from build123d import *

# Parameters (mm, degrees)
F0_W         = 156
F0_H         = 10
F0_R         = 1.5
F1_DEPTH     = 8
F2_T1_DEPTH  = 4
F2_T3_DEPTH  = 18
F2_T5_DEPTH  = 159
F2_T7_DEPTH  = 13
F2_S11_W     = 2
F2_S11_H     = 2
F2_T12_DEPTH = 2
F2_S17_W     = 2
F2_S17_H     = 2
F2_T18_DEPTH = 2
F3_T1_DEPTH  = 11
F3_T3_DEPTH  = 4
F3_T5_DEPTH  = 157
F3_S9_W      = 2.04
F3_S9_H      = 2.04
F3_T10_DEPTH = 2.04
F3_S15_W     = 2.04
F3_S15_H     = 2.04
F3_T16_DEPTH = 2.04


# Not quite as in the source:
# - a fillet or chamfer that OpenCascade refuses, or shapes differently, is made with other operations: its cross-section is extruded or revolved along the edge and cut away or added


with BuildPart() as f1:
    # F0 (on Front) → F1 (new body)
    with BuildSketch(Plane.XZ):
        with Locations((-25, 5)):
            Rectangle(F0_W, F0_H)
        with Locations((-100, 5)):
            Circle(F0_R, mode=Mode.SUBTRACT)
        with Locations((50, 5)):
            Circle(F0_R, mode=Mode.SUBTRACT)
    extrude(amount=F1_DEPTH)

    # F2: fillet of radius 2 on 7 edges, made by hand

    # F2_s2 → F2_t1 (cut)
    with BuildSketch(Plane.XZ.offset(2)):
        with BuildLine():
            ThreePointArc((53, 8), (52.4142135624, 9.4142135624), (51, 10))
            Line((51, 10), (53, 10))
            Line((53, 10), (53, 8))
        make_face()
    extrude(amount=F2_T1_DEPTH, mode=Mode.SUBTRACT)

    # F2_s4 → F2_t3 (cut)
    with BuildSketch(Plane.XZ.offset(-5)):
        with BuildLine():
            ThreePointArc((-103, 8), (-102.4142135624, 9.4142135624), (-101, 10))
            Line((-101, 10), (-103, 10))
            Line((-103, 10), (-103, 8))
        make_face()
        with BuildLine():
            ThreePointArc((51, 0), (52.4142135624, 0.5857864376), (53, 2))
            Line((53, 2), (53, 0))
            Line((53, 0), (51, 0))
        make_face()
    extrude(amount=F2_T3_DEPTH, mode=Mode.SUBTRACT)

    # F2_s6 → F2_t5 (cut)
    with BuildSketch(Plane.YZ.offset(-108)):
        with BuildLine():
            ThreePointArc((-2, 10), (-0.5857864376, 9.4142135624), (0, 8))
            Line((0, 8), (0, 10))
            Line((0, 10), (-2, 10))
        make_face()
        with BuildLine():
            ThreePointArc((-6, 10), (-7.4142135624, 9.4142135624), (-8, 8))
            Line((-8, 8), (-8, 10))
            Line((-8, 10), (-6, 10))
        make_face()
    extrude(amount=F2_T5_DEPTH, mode=Mode.SUBTRACT)

    # F2_s8 → F2_t7 (cut)
    with BuildSketch(Plane.XY.offset(-5)):
        with BuildLine():
            ThreePointArc((53, -2), (52.4142135624, -0.5857864376), (51, 0))
            Line((51, 0), (53, 0))
            Line((53, 0), (53, -2))
        make_face()
        with BuildLine():
            ThreePointArc((53, -6), (52.4142135624, -7.4142135624), (51, -8))
            Line((51, -8), (53, -8))
            Line((53, -8), (53, -6))
        make_face()
    extrude(amount=F2_T7_DEPTH, mode=Mode.SUBTRACT)


with BuildPart() as f2_tool10:
    # F2_s11 → F2_t12 (new body)
    with BuildSketch(Plane.YZ.offset(51)):
        with Locations((-1, 9)):
            Rectangle(F2_S11_W, F2_S11_H)
    extrude(amount=F2_T12_DEPTH)

    # F2_s13 → F2_t14 (revolve, cut)
    with BuildSketch(Plane(origin=(51, -2, 8), x_dir=(0, -0.7071067812, -0.7071067812), z_dir=(0, -0.7071067812, 0.7071067812))):
        with BuildLine():
            ThreePointArc((0, -2), (2, 0), (0, 2))
            Line((0, 2), (0, -2))
        make_face()
    revolve(axis=Axis((51, -2, 8), (1, 0, 0)), mode=Mode.SUBTRACT)


with BuildPart() as f1_1:
    add(f1.part)

    # F2_t9: cut F2_tool10
    add(f2_tool10.part, mode=Mode.SUBTRACT)


with BuildPart() as f2_tool16:
    # F2_s17 → F2_t18 (new body)
    with BuildSketch(Plane.YZ.offset(51)):
        with Locations((-7, 9)):
            Rectangle(F2_S17_W, F2_S17_H)
    extrude(amount=F2_T18_DEPTH)

    # F2_s19 → F2_t20 (revolve, cut)
    with BuildSketch(Plane(origin=(51, -6, 8), x_dir=(0, 0.7071067812, -0.7071067812), z_dir=(0, -0.7071067812, -0.7071067812))):
        with BuildLine():
            ThreePointArc((0, -2), (2, 0), (0, 2))
            Line((0, 2), (0, -2))
        make_face()
    revolve(axis=Axis((51, -6, 8), (1, 0, 0)), mode=Mode.SUBTRACT)


with BuildPart() as f1_2:
    add(f1_1.part)

    # F2_t15: cut F2_tool16
    add(f2_tool16.part, mode=Mode.SUBTRACT)

    # F3: fillet of radius 2 on 7 edges, made by hand

    # F3_s2 → F3_t1 (cut)
    with BuildSketch(Plane.XY.offset(2)):
        with BuildLine():
            ThreePointArc((-103, -2), (-102.4142135624, -0.5857864376), (-101, 0))
            Line((-101, 0), (-103, 0))
            Line((-103, 0), (-103, -2))
        make_face()
        with BuildLine():
            ThreePointArc((-103, -6), (-102.4142135624, -7.4142135624), (-101, -8))
            Line((-101, -8), (-103, -8))
            Line((-103, -8), (-103, -6))
        make_face()
    extrude(amount=F3_T1_DEPTH, mode=Mode.SUBTRACT)

    # F3_s4 → F3_t3 (cut)
    with BuildSketch(Plane.XZ.offset(2)):
        with BuildLine():
            ThreePointArc((-103, 2), (-102.4142135624, 0.5857864376), (-101, 0))
            Line((-101, 0), (-103, 0))
            Line((-103, 0), (-103, 2))
        make_face()
    extrude(amount=F3_T3_DEPTH, mode=Mode.SUBTRACT)

    # F3_s6 → F3_t5 (cut)
    with BuildSketch(Plane.YZ.offset(-101)):
        with BuildLine():
            ThreePointArc((0, 2), (-0.5857864376, 0.5857864376), (-2, 0))
            Line((-2, 0), (0, 0))
            Line((0, 0), (0, 2))
        make_face()
        with BuildLine():
            ThreePointArc((-6, 0), (-7.4142135624, 0.5857864376), (-8, 2))
            Line((-8, 2), (-8, 0))
            Line((-8, 0), (-6, 0))
        make_face()
    extrude(amount=F3_T5_DEPTH, mode=Mode.SUBTRACT)


with BuildPart() as f3_tool8:
    # F3_s9 → F3_t10 (new body)
    with BuildSketch(Plane.YZ.offset(-101)):
        with Locations((-0.98, 0.98)):
            Rectangle(F3_S9_W, F3_S9_H)
    extrude(amount=-F3_T10_DEPTH)

    # F3_s11 → F3_t12 (revolve, cut)
    with BuildSketch(Plane(origin=(-101, -2, 2), x_dir=(0, -0.7071067812, 0.7071067812), z_dir=(0, -0.7071067812, -0.7071067812))):
        with BuildLine():
            ThreePointArc((0, -2), (2, 0), (0, 2))
            Line((0, 2), (0, -2))
        make_face()
    revolve(axis=Axis((-101, -2, 2), (-1, 0, 0)), mode=Mode.SUBTRACT)


with BuildPart() as f1_3:
    add(f1_2.part)

    # F3_t7: cut F3_tool8
    add(f3_tool8.part, mode=Mode.SUBTRACT)


with BuildPart() as f3_tool14:
    # F3_s15 → F3_t16 (new body)
    with BuildSketch(Plane.YZ.offset(-101)):
        with Locations((-7.02, 0.98)):
            Rectangle(F3_S15_W, F3_S15_H)
    extrude(amount=-F3_T16_DEPTH)

    # F3_s17 → F3_t18 (revolve, cut)
    with BuildSketch(Plane(origin=(-101, -6, 2), x_dir=(0, 0.7071067812, 0.7071067812), z_dir=(0, -0.7071067812, 0.7071067812))):
        with BuildLine():
            ThreePointArc((0, -2), (2, 0), (0, 2))
            Line((0, 2), (0, -2))
        make_face()
    revolve(axis=Axis((-101, -6, 2), (-1, 0, 0)), mode=Mode.SUBTRACT)


with BuildPart() as f1_4:
    add(f1_3.part)

    # F3_t13: cut F3_tool14
    add(f3_tool14.part, mode=Mode.SUBTRACT)


solid = f1_4.part
Input: part model. Units: mm. Frame: model coordinates. Give positions to 0.01 mm unless a question says otherwise; leave off trailing zeros. Write each loop counter-clockwise with the first axis right and the second up, starting at its lowest first coordinate (ties: lowest second). Pieces come first, ordered by that corner, then holes. Notation, with made-up numbers: (80, -15) -> (120, -15) arc R30 cw to (120, 11) -> close; hole circle Ø9 at (-5.5, -18). An arc over 180 degrees is marked (long way). Use one line per item in the form item = value. Start each with the question number.
1) Section query A-A on x = -4.5. Return the cut outline in (y, z), then the cut area to 3 significant figures.
2) Ray query, probe 1 along X at (y, z) = (-5.25, 5.25); probe 2 along Z at (x, y) = (-100, -3); probe 3 along Z at (x, y) = (-52, -1.75). Return the intervals inside material, ascending. Write a range as from..to.
3) Draft query along X for faces 1 (the cylindrical face through (48.5, -3.94, 5.07)), 2 (the flat face through (-26, 0, 5)), 3 (the flat face through (-103, -4, 5)). Return one class per face: pulls with the +X half, pulls with the -X half, needs draft (parallel to the pull), parting line crosses it, or undercut.
Outcome:
q1.outline = (-8, 2) arc R2 ccw to (-6, 0) -> (-2, 0) arc R2 ccw to (0, 2) -> (0, 8) arc R2 ccw to (-2, 10) -> (-6, 10) arc R2 ccw to (-8, 8) -> close
q1.area = 76.6 mm^2
q2.probe_1 = -103..-101.48, -98.52..48.52, 51.48..53
q2.probe_2 = 0..3.5, 6.5..10
q2.probe_3 = 0.02..9.98
q3.face_1 = undercut
q3.face_2 = needs draft
q3.face_3 = pulls with the -X half
